Here's the drawing with two shaded views (mm, measured from the low corner). I have some questions. A direction names the side the tool comes from. Round coordinates to 2 decimals unless told otherwise and drop trailing zeros. Order: outer loops, then holes, each group sorted by start corner. A loop starts at its lowest first (then second) coordinate and runs counter-clockwise, first axis right, second up. Notation, with made-up numbers: M 31.5,39.5 L 71.5,39.5 A26 ccw 71.5,76.5 Z; hole C -26.75,-28 d6. An arc over 180 degrees is marked long. One line per question, with ' | ' between items.
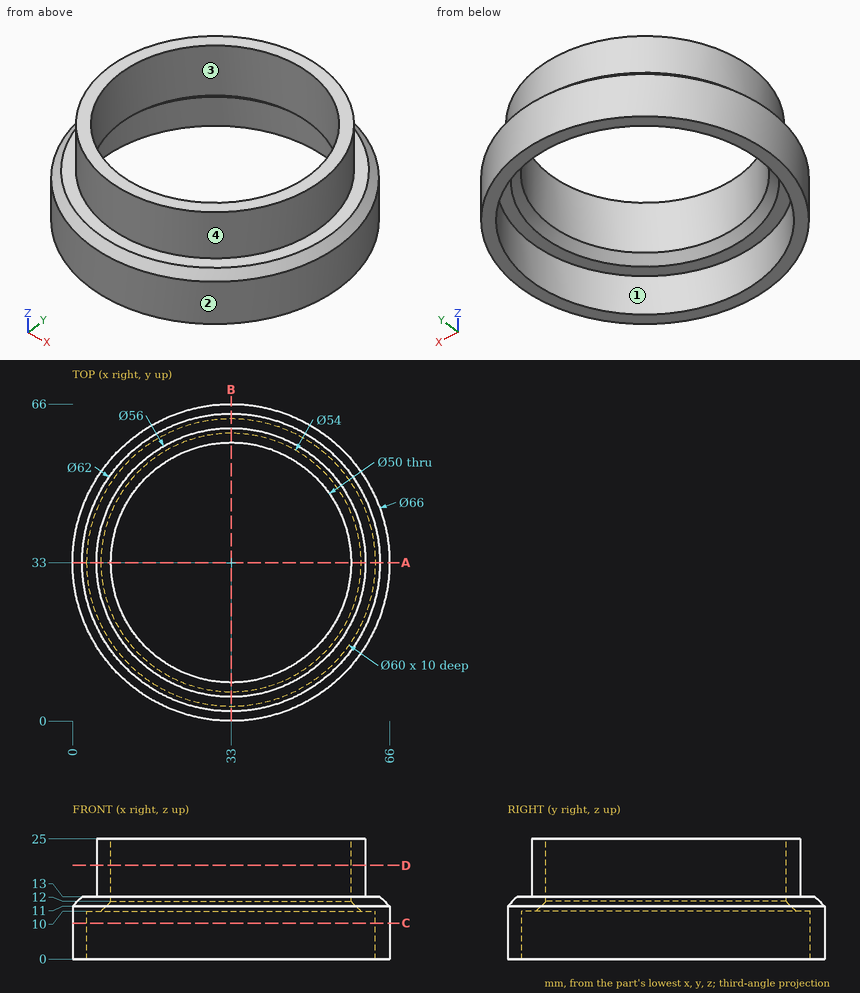
(1) If we section it at A-A on y = 33: Please give me the cut outline in (x, z), plus the area to 3 significant figures.
Final values:
outline: M 0,0 L 3,0 L 3,10 L 6,10 L 8,12 L 8,25 L 5,25 L 5,13 L 2,13 L 0,11 Z; M 58,12 L 60,10 L 63,10 L 63,0 L 66,0 L 66,11 L 64,13 L 61,13 L 61,25 L 58,25 Z | area: 172 mm^2
(2) If we section it at C-C on z = 7.5: Please give me the cut outline in (x, y).
Final values:
outline: C 33,33 d66; hole C 33,33 d60
(3) Thinking about a two-plate mould opening in X: for the marked faces 1 and 2, which applies, released by +X, released by -X, zero draft, split by the parting line, or undercut?
Final values:
face 1: undercut | face 2: split by the parting line
(4) On a 3-axis mill with a long thin cutter (end or side, diameter ignored), from which of +Z, -Z, +X, -X, +Y, -Y can I reach the whole of each face in a straight line? I mean the marked faces 3 and 4. Say none if no direction works.
Final values:
face 3: +Z, -Z | face 4: +Z
(5) Will these pins go through, and if not, where does the flat tip stop? pin 1 Ø12 at (y, z) = (29.5, 18) entering from +X; pin 2 Ø5 at (x, y) = (7, 34.5) entering from -Z; pin 3 Ø18 at (x, y) = (46, 33.5) entering from -Z; pin 4 Ø2 at (x, z) = (45.5, 8.5) entering from -Y.
Final values:
pin 1: x = 64.84 | pin 2: z = 10 | pin 3: through | pin 4: y = 2.07
(6) Please list where these lines run through material, in increasing order: probe 1 along Y at (x, z) = (33, 21.75); probe 2 along Y at (x, z) = (33, 5); probe 3 along X at (y, z) = (28, 2). Write a range as [from, to].
Final values:
probe 1: [5, 8], [58, 61] | probe 2: [0, 3], [63, 66] | probe 3: [0.38, 3.42], [62.58, 65.62]
(7) If we section it at D-D on z = 19.5: Please give me the cut outline in (x, y), plus the area to 3 significant figures.
Final values:
outline: C 33,33 d56; hole C 33,33 d50 | area: 500 mm^2
